Source: three-view drawing plus pictorial views. Frame: mm from the lowest corner of the part. Give positions to 0.01 mm unless a question says otherwise; leave off trailing zeros. Loops run counter-clockwise (first coordinate to the right, second up) from the corner with the lowest first, then second, coordinate; pieces in that order, holes last. Notation, with made-up numbers: (15.5, 89.5) -> (74.5, 89.5) arc R20 ccw to (74.5, 124.5) -> close; hole circle Ø4 at (47.25, 10). An arc over 180 degrees is marked (long way). One line per item, written item: value. Start each with the question number.
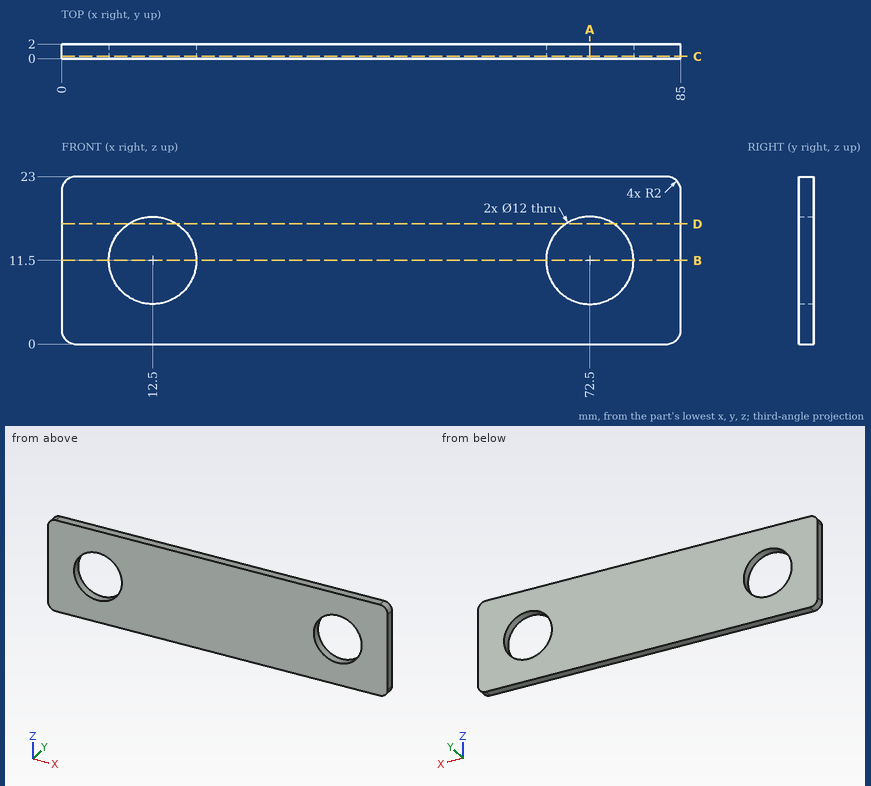
Item 1: Section B-B, the plane z = 11.5. Output: boundary loops of the cut face in (x, y).
Item 2: Section D-D, the plane z = 16.5. Output: boundary loops of the cut face in (x, y).
Item 3: Section C-C, the plane y = 0.3. Output: boundary loops of the cut face in (x, z), then the cut area to 3 significant figures.
Item 4: Section A-A, the plane x = 72.5. Output: boundary loops of the cut face in (y, z).
Item 5: Ray query, line 1 along X through (y, z) = (1.15, 11.5); line 2 along Z through (x, y) = (72.5, 1.05); line 3 along X through (y, z) = (0.25, 6.5). Return the intervals inside material, ascending. Write a range as [from, to].
Geometry check:
1. outline: (0, 0) -> (6.5, 0) -> (6.5, 2) -> (0, 2) -> close; (18.5, 0) -> (66.5, 0) -> (66.5, 2) -> (18.5, 2) -> close; (78.5, 0) -> (85, 0) -> (85, 2) -> (78.5, 2) -> close
2. outline: (0, 0) -> (9.18, 0) -> (9.18, 2) -> (0, 2) -> close; (15.82, 0) -> (69.18, 0) -> (69.18, 2) -> (15.82, 2) -> close; (75.82, 0) -> (85, 0) -> (85, 2) -> (75.82, 2) -> close
3. outline: (0, 2) arc R2 ccw to (2, 0) -> (83, 0) arc R2 ccw to (85, 2) -> (85, 21) arc R2 ccw to (83, 23) -> (2, 23) arc R2 ccw to (0, 21) -> close; hole circle Ø12 at (12.5, 11.5); hole circle Ø12 at (72.5, 11.5)
3. area: 1,730 mm2
4. outline: (0, 0) -> (2, 0) -> (2, 5.5) -> (0, 5.5) -> close; (0, 17.5) -> (2, 17.5) -> (2, 23) -> (0, 23) -> close
5. line 1: x = [0, 6.5], [18.5, 66.5], [78.5, 85]
5. line 2: z = [0, 5.5], [17.5, 23]
5. line 3: x = [0, 9.18], [15.82, 69.18], [75.82, 85]
